Geometry check sheet. Reference: the model listing, model coordinates, mm. A direction names the side the tool comes from. Give positions to 0.01 mm unless a question says otherwise; leave off trailing zeros. Loops run counter-clockwise (first coordinate to the right, second up) from the corner with the lowest first, then second, coordinate; pieces in that order, holes last. Notation, with made-up numbers: (12, 24.25) - (69, 24.25) arc R24 cw to (69, 36.25) - close; hole circle Ø2 at (-20.5, 80). An arc over 180 degrees is marked (long way). One line per question, with ' | ' between items. Start each with the question number.
from build123d import *

# Parameters (mm, degrees)
F0_R     = 31.5
F0_R_2   = 3.45
F1_DEPTH = 2
F2_R     = 2.5
F3_DEPTH = 40
F4_SIZE2 = 9.3301270189
F4_SIZE  = 2.5


with BuildPart() as f1:
    # F0 (on Top) → F1 (new body)
    with BuildSketch(Plane.XY):
        Circle(F0_R)
        with Locations((-16.5, 0)):
            Circle(F0_R_2, mode=Mode.SUBTRACT)
        with Locations((16.5, 0)):
            Circle(F0_R_2, mode=Mode.SUBTRACT)
    extrude(amount=F1_DEPTH)

    # F2 (on face) → F3 (join)
    with BuildSketch(Plane.XY.offset(2)):
        Circle(F2_R)
    extrude(amount=F3_DEPTH)

    # F4
    f4_edges = [f1.edges().sort_by_distance(p)[0] for p in [
        (-2.5, 0, 42),
    ]]
    f4_side = f1.faces().sort_by_distance((0, 0, 42))[0]
    chamfer(f4_edges, length=F4_SIZE, length2=F4_SIZE2, reference=f4_side)


solid = f1.part
(1) Mould release check, pull along X, two halves, no side actions. Record for faces 3 (the face through (-19.947, 0.152, 0.986)), 4 (the face through (-4.101, 31.232, 0.986)), 5 (the face through (7, 0, 2)): pulls with the +X half, pulls with the -X half, needs draft (parallel to the pull), parting line crosses it, or undercut.
(2) Section check B-B, the plane z = 31. Record the boundary of the cut face in (x, y), and give its area (3 significant figures).
(3) Material ranges on line 1 (Z direction, x = -17.5, y = 24.5); line 2 (Y direction, x = 16.5, z = 1.05); line 3 (Y direction, x = -16, z = 1), recorded low to high.
(4) Tool access check on faces 1 (the face through (-0.54, -2.44, 17.12)), 2 (the face through (0, 0, 0)). Record the directions out of +Z, -Z, +X, -X, +Y, -Y that give a thin tool (end or side, any length) a straight path to the whole face; none if there is none.
(5) Section check C-C, the plane y = -7. Record the boundary of the cut face in (x, z).
(6) Section check A-A, the plane x = -18.5. Record the boundary of the cut face in (y, z).
(7) Depth check by flat-ended pin: pin 1 Ø1.5 at (y, z) = (1.5, 34) entering from +X; pin 2 Ø5 at (x, y) = (-20, -16.5) entering from +Z; pin 3 Ø4 at (x, y) = (6.5, 4) entering from -Z; pin 4 Ø12 at (y, z) = (23.5, 7) entering from +X. Enter the tip coordinate at first touch or a pass-through.
(8) Section check D-D, the plane x = 8.5. Record the boundary of the cut face in (y, z), and give its area (3 significant figures).
Numbers:
1) face 3: undercut | face 4: parting line crosses it | face 5: needs draft
2) outline: circle Ø5 at (0, 0) | area: 19.6 mm^2
3) line 1: 0 to 2 | line 2: -26.83 to -3.45, 3.45 to 26.83 | line 3: -27.13 to -3.41, 3.41 to 27.13
4) face 1: +Z | face 2: -Z, +X, -X, +Y, -Y
5) outline: (-30.71, 0) - (30.71, 0) - (30.71, 2) - (-30.71, 2) - close
6) outline: (-25.5, 0) - (-2.81, 0) - (-2.81, 2) - (-25.5, 2) - close; (2.81, 0) - (25.5, 0) - (25.5, 2) - (2.81, 2) - close
7) pin 1: x = 2.08 | pin 2: z = 2 | pin 3: z = 0 | pin 4: x = 24.18
8) outline: (-30.33, 0) - (30.33, 0) - (30.33, 2) - (-30.33, 2) - close | area: 121 mm^2
